Work out the finished part from the listing and answer in its coordinate system (mm). A direction names the side the tool comes from. Give positions to 0.01 mm unless a question says otherwise; leave off trailing zeros. Loops run counter-clockwise (first coordinate to the right, second up) from the corner with the lowest first, then second, coordinate; pieces in that order, holes last. Notation, with made-up numbers: (82.5, -4) - (99.5, -4) arc R25 ccw to (99.5, 21) - close; hole circle Ø10 at (75.5, 13). An arc over 180 degrees is marked (long way). One line per question, with ' | ' between items.
from build123d import *

# Parameters (mm, degrees)
ESQUISSE1_W        = 30
ESQUISSE1_H        = 15
ESQUISSE1_R        = 2.5
BOSS_EXTRU_2_DEPTH = 5
ESQUISSE2_W        = 10
ESQUISSE2_H        = 15
BOSS_EXTRU_3_DEPTH = 10
BOSS_EXTRU_5_DEPTH = 25
CONG_1_R           = 10
CONG_2_R           = 3


with BuildPart() as part:
    # Esquisse1 → Boss.-Extru.2 (new body)
    with BuildSketch(Plane.XY):
        Rectangle(ESQUISSE1_W, ESQUISSE1_H)
        with Locations((-10, 0)):
            Circle(ESQUISSE1_R, mode=Mode.SUBTRACT)
        with Locations(Location((10, 0, 0), (0, 0, 180))):
            Circle(ESQUISSE1_R, mode=Mode.SUBTRACT)
    extrude(amount=BOSS_EXTRU_2_DEPTH)

    # Esquisse2 → Boss.-Extru.3 (add)
    with BuildSketch(Plane.XY.offset(5)):
        Rectangle(ESQUISSE2_W, ESQUISSE2_H)
    extrude(amount=BOSS_EXTRU_3_DEPTH)

    # Esquisse3 → Boss.-Extru.5 (add)
    with BuildSketch(Plane(origin=(0, 7.5, 0), x_dir=(1, 0, 0), z_dir=(0, 1, 0))):
        with BuildLine():
            ThreePointArc((5, -8), (0, -6.397674733), (-5, -8))
            Line((-5, -8), (-5, -15))
            Line((-5, -15), (5, -15))
            Line((5, -15), (5, -8))
        make_face()
    extrude(amount=BOSS_EXTRU_5_DEPTH)

    # Congé1
    cong_1_edges = [part.edges().sort_by_distance(p)[0] for p in [
        (0, -7.5, 15),
    ]]
    fillet(cong_1_edges, radius=CONG_1_R)

    # Congé2
    cong_2_edges = [part.edges().sort_by_distance(p)[0] for p in [
        (-5, 17.5, 15),
        (0, 32.5, 15),
        (5, 17.5, 15),
        (5, -4.571067812, 12.071067812),
        (-5, -4.571067812, 12.071067812),
    ]]
    fillet(cong_2_edges, radius=CONG_2_R)


solid = part.part
1. Find section A-A on x = -10. Write down the section's boundary in (y, z), then the cut area to 3 significant figures.
Evaluation:
outline: (-7.5, 0) - (-2.5, 0) - (-2.5, 5) - (-7.5, 5) - close; (2.5, 0) - (7.5, 0) - (7.5, 5) - (2.5, 5) - close | area: 50.0 mm2
2. Flat-ended cylindrical pins translate along their axes: pin 1 (12 mm diameter, centred on x = -8.5, y = 14.5, fed in from +Z); pin 2 (6 mm diameter, centred on x = -10, y = 0, fed in from +Z); pin 3 (5.5 mm diameter, centred on y = 18.5, z = 9.5, fed in from +X). Find the tip coordinate at first contact, or state that the pin passes through.
Evaluation:
pin 1: z = 14.96 | pin 2: z = 5 | pin 3: x = 5
3. Find section B-B on z = 4.5. Write down the section's boundary in (x, y).
Evaluation:
outline: (-15, -7.5) - (15, -7.5) - (15, 7.5) - (-15, 7.5) - close; hole circle Ø5 at (-10, 0); hole circle Ø5 at (10, 0)
4. Find section D-D on x = 13. Write down the section's boundary in (y, z).
Evaluation:
outline: (-7.5, 0) - (7.5, 0) - (7.5, 5) - (-7.5, 5) - close
5. Which of the six approach directions +Z, -Z, +X, -X, +Y, -Y give full straight-line access (tool end or side, diameter ignored) to faces 1 (the cylindrical face through (0.1, 19.8, 6.4)), 2 (the flat face through (5, 14, 9)), 3 (the flat face through (-5, 14, 9))?
Evaluation:
face 1: -Z, +Y | face 2: +Z, +X, +Y, -Y | face 3: +Z, -X, +Y, -Y
6. Find section C-C on y = 26. Write down the section's boundary in (x, z).
Evaluation:
outline: (-5, 8) arc R8.6 ccw to (5, 8) - (5, 12) arc R3 ccw to (2, 15) - (-2, 15) arc R3 ccw to (-5, 12) - close
7. Consider L1, parallel to Y at x = -10, z = 1.65; L2, parallel to X at y = 3.5, z = 7.5; L3, parallel to Z at x = -5.25, y = 4. Determine where each line is inside the solid, lowest interval first.
Evaluation:
L1: -7.5 to -2.5, 2.5 to 7.5 | L2: -5 to 5 | L3: 0 to 5
